The listing builds one solid part. Answer for the finished solid, in the listing's coordinates (mm). A direction names the side the tool comes from. Round coordinates to 2 decimals unless told otherwise and drop trailing zeros. Write each loop counter-clockwise with the first axis right and the second up, starting at its lowest first coordinate (ties: lowest second). Pieces come first, ordered by that corner, then holes. Notation, with made-up numbers: (-30.5, 6.25) - (6.5, 6.25) arc R27 cw to (6.5, 42.25) - close; hole circle Ø5 at (38.5, 84.5). An arc over 180 degrees is marked (long way). Answer in a Markdown table with one row per item.
Autodesk Fusion 360 part; units mm, degrees
sketch "Sketch1" plane through (0, 0, 0) normal (0, 0, 1) x (1, 0, 0)
  line L0 (0, 0) -> (43, 0)
  line L1 (43, 0) -> (43, 177.8)
  line L2 (43, 177.8) -> (0, 177.8)
  line L3 (0, 177.8) -> (0, 0)
  line L4 (0, 112.616) -> (-19.05, 112.616)
  line L5 (-19.05, 112.616) -> (-19.05, 102.616)
  line L6 (-19.05, 102.616) -> (0, 102.616)
  line L7 (0, 102.616) -> (0, 112.616)
  line L8 (43, 112.616) -> (62.05, 112.616)
  line L9 (62.05, 112.616) -> (62.05, 102.616)
  line L10 (62.05, 102.616) -> (43, 102.616)
  line L11 (43, 102.616) -> (43, 112.616)
  dimension "d1" = 177.8
  dimension "d2" = 43
  dimension "d5" = 75.184
  dimension "d6" = 75.184
  dimension "d7" = 10
  dimension "d8" = 10
  dimension "d9" = 19.05
  dimension "d10" = 19.05
extrude "Extrude1" add sketch "Sketch1" along normal blind 12.6
sketch "Sketch2" plane through (0, 0, 12.6) normal (0, 0, 1) x (-1, 0, 0)
  line L0 (-43, -112.616) -> (-43, -177.8)
  line L1 (-43, -177.8) -> (0, -177.8)
  line L2 (0, -177.8) -> (0, -112.616)
  line L3 (0, -112.616) -> (19.05, -112.616)
  line L4 (19.05, -112.616) -> (19.05, -102.616)
  line L5 (19.05, -102.616) -> (0, -102.616)
  line L6 (0, -102.616) -> (0, 0)
  line L7 (0, 0) -> (-43, 0)
  line L8 (-43, 0) -> (-43, -102.616)
  line L9 (-43, -102.616) -> (-62.05, -102.616)
  line L10 (-62.05, -102.616) -> (-62.05, -112.616)
  line L11 (-62.05, -112.616) -> (-43, -112.616)
  line L12 (-2, -102.616) -> (-41, -102.616)
  line L13 (-41, -102.616) -> (-41, -2)
  line L14 (-41, -2) -> (-2, -2)
  line L15 (-2, -2) -> (-2, -102.616)
  dimension "d11" = 2
  dimension "d12" = 2
  dimension "d13" = 2
  dimension "d20" = 10
extrude "Extrude2" cut sketch "Sketch2" against normal blind 10.6 contours L12 L13 L14 L15
sketch "Sketch4" plane through (0, 0, 12.6) normal (0, 0, 1) x (-1, 0, 0)
  line L0 (-41, -102.616) -> (-41, -2)
  line L1 (-41, -2) -> (-2, -2)
  line L2 (-2, -2) -> (-2, -102.616)
  line L3 (-2, -102.616) -> (-41, -102.616)
  line L4 (-43, -112.616) -> (-43, -177.8)
  line L5 (-43, -177.8) -> (0, -177.8)
  line L6 (0, -177.8) -> (0, -112.616)
  line L7 (0, -112.616) -> (19.05, -112.616)
  line L8 (19.05, -112.616) -> (19.05, -102.616)
  line L9 (19.05, -102.616) -> (0, -102.616)
  line L10 (0, -102.616) -> (0, 0)
  line L11 (0, 0) -> (-43, 0)
  line L12 (-43, 0) -> (-43, -102.616)
  line L13 (-43, -102.616) -> (-62.05, -102.616)
  line L14 (-62.05, -102.616) -> (-62.05, -112.616)
  line L15 (-62.05, -112.616) -> (-43, -112.616)
  line L16 (0, -102.616) -> (-43, -102.616)
  line L17 (-43, -102.616) -> (-43, 0)
  line L18 (-43, 0) -> (0, 0)
  line L19 (0, 0) -> (0, -102.616)
extrude "Extrude3" cut sketch "Sketch4" against normal blind 3 contours L0 L1 L2 L10 L11 L12 L16 L17 L18 L19
sketch "Sketch5" plane through (0, 177.8, 0) normal (0, 1, 0) x (-1, 0, 0)
  line L0 (-43, 0) -> (0, 0)
  line L1 (0, 0) -> (0, 12.6)
  line L2 (0, 12.6) -> (-43, 12.6)
  line L3 (-43, 12.6) -> (-43, 0)
  circle A0 centre (-21.5, 6.3) radius 2.7
  dimension "d21" = 5.4
  dimension "d22" = 6.3
extrude "Extrude4" cut sketch "Sketch5" against normal blind 83.82 contours A0
sketch "Sketch6" plane through (0, 0, 2) normal (0, 0, 1) x (-1, 0, 0)
  line L0 (-2, -2) -> (-41, -2)
  line L1 (-41, -2) -> (-41, -102.616)
  line L2 (-41, -102.616) -> (-2, -102.616)
  line L3 (-2, -102.616) -> (-2, -2)
  line L4 (-20.5, -102.616) -> (-22.5, -102.616)
  line L5 (-22.5, -102.616) -> (-22.5, -2)
  line L6 (-22.5, -2) -> (-20.5, -2)
  line L7 (-20.5, -2) -> (-20.5, -102.616)
  line L8 (-43, -102.616) -> (-43, 0)
  line L9 (-2, -52.308) -> (-41, -52.308)
  line L10 (-41, -52.308) -> (-41, -50.308)
  line L11 (-41, -50.308) -> (-2, -50.308)
  line L12 (-2, -50.308) -> (-2, -52.308)
  line L13 (-43, 0) -> (0, 0)
  dimension "d25" = 2
  dimension "d26" = 20.5
  dimension "d27" = 2
  dimension "d28" = 50.308
extrude "Extrude5" cut sketch "Sketch6" against normal blind 0.4 contours L0 L5 L6 L7 L11 | L3 L7 L9 L11 L12 | L5 L7 L9 L11 | L1 L5 L9 L10 L11 | L2 L4 L5 L7 L9
sketch "Sketch7" plane through (0, 112.616, 0) normal (0, 1, 0) x (-1, 0, 0)
  line L0 (0, 0) -> (19.05, 0)
  line L1 (19.05, 0) -> (19.05, 12.6)
  line L2 (19.05, 12.6) -> (0, 12.6)
  line L3 (0, 12.6) -> (0, 0)
  circle A0 centre (9.705, 6.3) radius 1.4986
  circle A1 centre (-52.7028, 6.3) radius 1.4986
  line L4 (-43, 0) -> (-43, 12.6)
  dimension "d31" = 2.9972
  dimension "d32" = 2.9972
  dimension "d33" = 62.4078
  dimension "d34" = 9.7028
extrude "Extrude6" cut sketch "Sketch7" against normal blind 12.7 contours A0 | A1
(1) Flat-ended cylindrical pins translate along their axes: pin 1 (20.5 mm diameter, centred on x = 33.5, y = 32, fed in from +Z); pin 2 (15 mm diameter, centred on x = 30.5, y = 82.5, fed in from +Z); pin 3 (4 mm diameter, centred on y = 31.5, z = 9, fed in from -X). Find the tip coordinate at first contact, or state that the pin passes through.
Checked values:
| item | result |
|---|---|
| pin 1 | stops at z = 9.6 |
| pin 2 | stops at z = 2 |
| pin 3 | stops at x = 0 |
(2) Section B-B (x = 14) is taken. Give the vertices of the cut face in (y, z).
Checked values:
| item | result |
|---|---|
| outline | (0, 0) - (177.8, 0) - (177.8, 12.6) - (102.62, 12.6) - (102.62, 2) - (52.31, 2) - (52.31, 1.6) - (50.31, 1.6) - (50.31, 2) - (2, 2) - (2, 9.6) - (0, 9.6) - close |
(3) Section A-A (y = 46.5) is taken. Give the vertices of the cut face in (x, z).
Checked values:
| item | result |
|---|---|
| outline | (0, 0) - (43, 0) - (43, 9.6) - (41, 9.6) - (41, 2) - (22.5, 2) - (22.5, 1.6) - (20.5, 1.6) - (20.5, 2) - (2, 2) - (2, 9.6) - (0, 9.6) - close |
(4) Find the intervals of material crossed by line 1 (X direction, y = 65, z = 4.75); line 2 (Y direction, x = 14.5, z = 3); line 3 (Y direction, x = 22, z = 5.25), in increasing order.
Checked values:
| item | result |
|---|---|
| line 1 | x = 0 to 2, 41 to 43 |
| line 2 | y = 0 to 2, 102.62 to 177.8 |
| line 3 | y = 0 to 2 |
(5) For a pull along Z with two mould halves and no side action, classify faces 1 (the flat face through (41, 53, 6)), 2 (the cylindrical face through (51.273, 107.686, 6.75)), 3 (the cylindrical face through (18.925, 140.734, 7.111)), 4 (the flat face through (21, 141, 12.6)) as pulls with the +Z half, pulls with the -Z half, needs draft (parallel to the pull), parting line crosses it, or undercut.
Checked values:
| item | result |
|---|---|
| face 1 | needs draft |
| face 2 | undercut |
| face 3 | undercut |
| face 4 | pulls with the +Z half |
(6) For faces 5 (the flat face through (1, 36, 9.6)), 6 (the flat face through (0, 52, 5)), 7 (the flat face through (-12, 112.616, 6)), 8 (the flat face through (43, 145, 6)), 9 (the flat face through (22, 2, 6)), determine the directions among +Z, -Z, +X, -X, +Y, -Y from which every point of the face is accessible in a straight line to the end or side of a thin tool.
Checked values:
| item | result |
|---|---|
| face 5 | +Z, +X, -X, -Y |
| face 6 | +Z, -Z, -X, -Y |
| face 7 | +Z, -Z, -X, +Y |
| face 8 | +Z, -Z, +X, +Y |
| face 9 | +Z |
